Can you work these out from the drawing? Everything is in mm from the part's minimum corner. Round coordinates to 2 decimals unless told otherwise and drop trailing zeros. Loops run counter-clockwise (first coordinate to the right, second up) from the corner with the lowest first, then second, coordinate; pieces in that order, holes last. Notation, with made-up numbers: (-38, 40) - (-10, 40) arc R12 cw to (-10, 45) - close; hole circle Ø11 at (56, 84.25). An arc over 180 degrees is marked (long way). Answer as a JSON object with one key per item and string values. Group by question number.
1) If I drill on line 1 along X through (y, z) = (26, 1.75); line 2 along Y through (x, z) = (19, 0.35) (1 decimal); line 3 along X through (y, z) = (144, 2.2) (1 decimal), over which ranges is the centre line in solid material (lowest first)? Write a range as [from, to].
2) If we mould it in two halves opening along Z, with no side actions, what happens to the marked faces 1 and 2? For each: pulls with the +Z half, pulls with the -Z half, needs draft (parallel to the pull), parting line crosses it, or undercut.
3) I want a section at A-A, the plane z = 0.7. Please give me the cut outline in (x, y) (1 decimal), then the cut area to 3 significant figures.
4) Will these pins go through, and if not, where does the flat tip stop? P1, Ø1.5, axis at y = 94.5, z = 2, coming from the -X side; P2, Ø1, axis at y = 52.5, z = 1, coming from the -X side.
5) I want a section at B-B, the plane y = 118. Please give me the cut outline in (x, z).
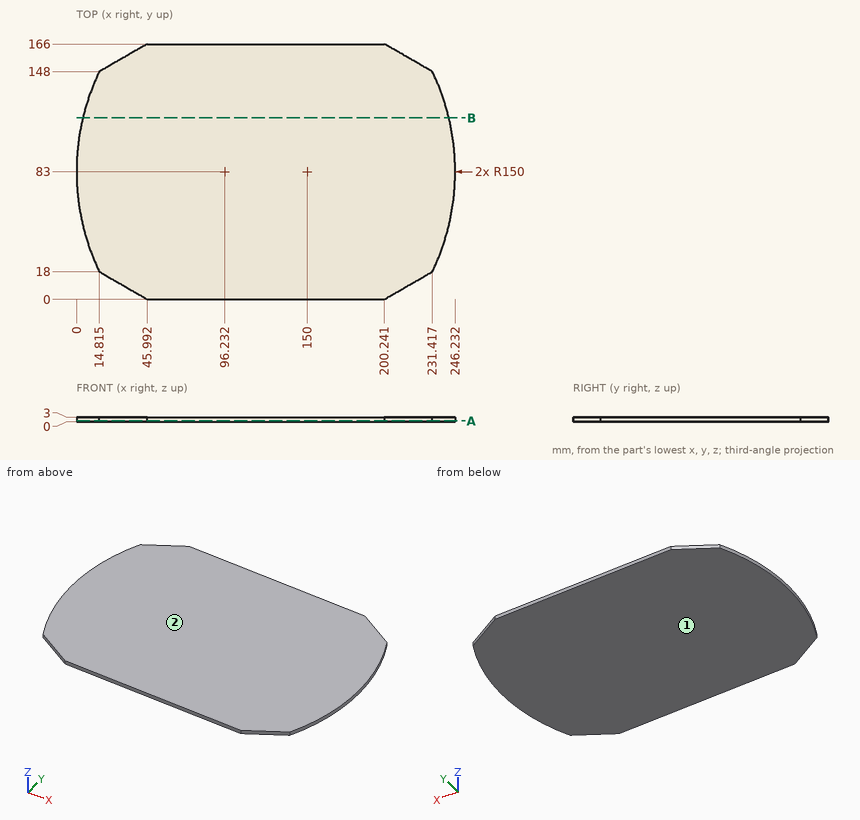
Outcome:
{
 "1": {"line 1": "[11.25, 234.98]", "line 2": "[15.6, 150.4]", "line 3": "[13, 233.3]"},
 "2": {"face 1": "pulls with the -Z half", "face 2": "pulls with the +Z half"},
 "3": {"outline": "(14.8, 18) - (46, 0) - (200.2, 0) - (231.4, 18) arc R150 ccw to (231.4, 148) - (200.2, 166) - (46, 166) - (14.8, 148) arc R150 ccw to start", "area": "37,400 mm^2"},
 "4": {"P1": "x = 0.39", "P2": "x = 3.03"},
 "5": {"outline": "(4.14, 0) - (242.09, 0) - (242.09, 3) - (4.14, 3) - close"}
}
